Source: CAD feature listing. Evaluate the final solid. Frame: model axes, mm. Face numbers are marked on the shaded views. A direction names the side the tool comes from. Coordinates: 2 decimals unless noted, no trailing zeros. Order: outer loops, then holes, each group sorted by start corner. A loop starts at its lowest first (then second) coordinate and runs counter-clockwise, first axis right, second up.
Item 1: Section A-A on y = 0. Return the cut outline in (x, z).
Item 2: Reachability of the marked faces 1 and 2 from +Z, -Z, +X, -X, +Y, -Y: full face, straight path, thin tool, end or side. Return the list, or none.
Item 3: Mould query, pull axis Y, two halves, no side actions, for the marked faces 3 and 4. Classes: released by +Y, released by -Y, zero draft, split by the parting line, or undercut.
Item 4: Ray query, line 1 (Y direction, x = 2.5, z = 1.25); line 2 (Y direction, x = 0, z = -5.5); line 3 (X direction, y = 6.75, z = 5). Return the intervals inside material, ascending.
Item 5: Contact query for a flat-ended pin moving along its axis: P1, Ø1, axis at y = -1.5, z = -8, coming from the -X side. Output: stop coordinate, or through.
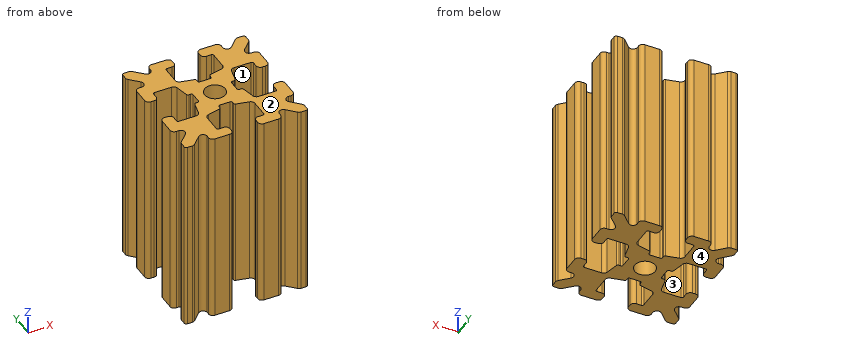
from build123d import *

# Parameters (mm, degrees)
SKETCH1_W           = 15
SKETCH1_H           = 15
SKETCH1_R           = 1.25
BOSS_EXTRUDE1_DEPTH = 12
FILLET1_R           = 0.25
CUT_EXTRUDE1_DEPTH  = 25
CUT_EXTRUDE3_DEPTH  = 25
FILLET3_R           = 0.5
FILLET4_R           = 0.5
FILLET5_R           = 3
FILLET6_R           = 0.2
CUT_EXTRUDE4_DEPTH  = 25
FILLET8_R           = 0.5
SKETCH6_W           = 5.1529354
SKETCH6_H           = 1.651
SKETCH6_W_2         = 1.651
SKETCH6_H_2         = 5.1529354
CUT_EXTRUDE5_DEPTH  = 25
FILLET10_R          = 0.2


with BuildPart() as part:
    # Sketch1 → Boss-Extrude1 (new body, symmetric)
    with BuildSketch(Plane.XY):
        Rectangle(SKETCH1_W, SKETCH1_H)
        Circle(SKETCH1_R, mode=Mode.SUBTRACT)
    extrude(amount=BOSS_EXTRUDE1_DEPTH, both=True)

    # Fillet1
    fillet1_edges = [part.edges().sort_by_distance(p)[0] for p in [
        (7.5, -7.5, 0),
        (-7.5, -7.5, 0),
        (-7.5, 7.5, 0),
        (7.5, 7.5, 0),
    ]]
    fillet(fillet1_edges, radius=FILLET1_R)

    # Sketch2 → Cut-Extrude1 (cut, through all)
    with BuildSketch(Plane.XY.offset(12)):
        Polygon((-7.5, 1.6), (-6.1, 1.6), (-6.1, 2.9), (-3.4, 2.9), (-3.4, -2.9), (-6.1, -2.9), (-6.1, -1.6), (-7.5, -1.6), align=None)
        Polygon((2.9, 6.1), (1.6, 6.1), (1.6, 7.5), (-1.6, 7.5), (-1.6, 6.1), (-2.9, 6.1), (-2.9, 3.4), (2.9, 3.4), align=None)
        Polygon((-1.6, -7.5), (-1.6, -6.1), (-2.9, -6.1), (-2.9, -3.4), (2.9, -3.4), (2.9, -6.1), (1.6, -6.1), (1.6, -7.5), align=None)
        Polygon((6.1, -2.9), (6.1, -1.6), (7.5, -1.6), (7.5, 1.6), (6.1, 1.6), (6.1, 2.9), (3.4, 2.9), (3.4, -2.9), align=None)
    extrude(amount=-CUT_EXTRUDE1_DEPTH, mode=Mode.SUBTRACT)

    # Sketch4 → Cut-Extrude3 (cut, through all)
    with BuildSketch(Plane.XY.offset(12)):
        Polygon((-3.4, 2.9), (-2.75, 0), (-3.4, -2.9), align=None)
        Polygon((-2.9, 3.4), (0, 2.75), (2.9, 3.4), align=None)
        Polygon((3.4, 2.9), (2.75, 0), (3.4, -2.9), align=None)
        Polygon((-2.9, -3.4), (0, -2.75), (2.9, -3.4), align=None)
    extrude(amount=-CUT_EXTRUDE3_DEPTH, mode=Mode.SUBTRACT)

    # Fillet3
    fillet3_edges = [part.edges().sort_by_distance(p)[0] for p in [
        (1.6, -7.5, 0),
        (-1.6, -7.5, 0),
        (-1.6, -6.1, 0),
        (1.6, -6.1, 0),
        (6.1, 1.6, 0),
        (7.5, 1.6, 0),
        (7.5, -1.6, 0),
        (6.1, -1.6, 0),
        (-7.5, -1.6, 0),
        (-7.5, 1.6, 0),
        (-6.1, 1.6, 0),
        (-6.1, -1.6, 0),
        (-1.6, 6.1, 0),
        (-1.6, 7.5, 0),
        (1.6, 7.5, 0),
        (1.6, 6.1, 0),
    ]]
    fillet(fillet3_edges, radius=FILLET3_R)

    # Fillet4
    fillet4_edges = [part.edges().sort_by_distance(p)[0] for p in [
        (-2.9, -3.4, 0),
        (2.9, -3.4, 0),
        (3.4, -2.9, 0),
        (3.4, 2.9, 0),
        (-3.4, 2.9, 0),
        (-3.4, -2.9, 0),
        (2.9, 3.4, 0),
        (-2.9, 3.4, 0),
    ]]
    fillet(fillet4_edges, radius=FILLET4_R)

    # Fillet5
    fillet5_edges = [part.edges().sort_by_distance(p)[0] for p in [
        (-2.75, 0, 0),
        (0, 2.75, 0),
        (2.75, 0, 0),
        (0, -2.75, 0),
    ]]
    fillet(fillet5_edges, radius=FILLET5_R)

    # Fillet6
    fillet6_edges = [part.edges().sort_by_distance(p)[0] for p in [
        (-2.9, -6.1, 0),
        (2.9, -6.1, 0),
        (6.1, -2.9, 0),
        (6.1, 2.9, 0),
        (-6.1, 2.9, 0),
        (-6.1, -2.9, 0),
        (2.9, 6.1, 0),
        (-2.9, 6.1, 0),
    ]]
    fillet(fillet6_edges, radius=FILLET6_R)

    # Sketch5 → Cut-Extrude4 (cut, through all)
    with BuildSketch(Plane.XY.offset(12)):
        Polygon((-7.5, 6.439339828), (-5.460660172, 4.4), (-7.5, 4.4), align=None)
        Polygon((-6.439339828, 7.5), (-4.4, 5.460660172), (-4.4, 7.5), align=None)
        Polygon((4.4, 7.5), (6.439339828, 7.5), (4.4, 5.460660172), align=None)
        Polygon((7.5, 6.439339828), (7.5, 4.4), (5.460660172, 4.4), align=None)
        Polygon((7.5, -6.439339828), (5.460660172, -4.4), (7.5, -4.4), align=None)
        Polygon((6.439339828, -7.5), (4.4, -5.460660172), (4.4, -7.5), align=None)
        Polygon((-4.4, -7.5), (-6.439339828, -7.5), (-4.4, -5.460660172), align=None)
        Polygon((-7.5, -6.439339828), (-7.5, -4.4), (-5.460660172, -4.4), align=None)
    extrude(amount=-CUT_EXTRUDE4_DEPTH, mode=Mode.SUBTRACT)

    # Fillet8
    fillet8_edges = [part.edges().sort_by_distance(p)[0] for p in [
        (-7.5, 4.4, 0),
        (-7.5, 6.439339828, 0),
        (-5.460660172, 4.4, 0),
        (7.5, -4.4, 0),
        (7.5, -6.439339828, 0),
        (5.460660172, -4.4, 0),
        (5.460660172, 4.4, 0),
        (7.5, 6.439339828, 0),
        (7.5, 4.4, 0),
        (-4.4, 7.5, 0),
        (-4.4, 5.460660172, 0),
        (-6.439339828, 7.5, 0),
        (-5.460660172, -4.4, 0),
        (-7.5, -6.439339828, 0),
        (-7.5, -4.4, 0),
        (4.4, 5.460660172, 0),
        (4.4, 7.5, 0),
        (6.439339828, 7.5, 0),
        (6.439339828, -7.5, 0),
        (4.4, -7.5, 0),
        (4.4, -5.460660172, 0),
        (-6.439339828, -7.5, 0),
        (-4.4, -5.460660172, 0),
        (-4.4, -7.5, 0),
    ]]
    fillet(fillet8_edges, radius=FILLET8_R)

    # Sketch6 → Cut-Extrude5 (cut, through all)
    with BuildSketch(Plane.XY.offset(12)):
        with Locations((4.9235323, 0)):
            Rectangle(SKETCH6_W, SKETCH6_H)
        with Locations((0, -4.9235323)):
            Rectangle(SKETCH6_W_2, SKETCH6_H_2)
        with Locations((-4.9235323, 0)):
            Rectangle(SKETCH6_W, SKETCH6_H)
        with Locations((0, 4.9235323)):
            Rectangle(SKETCH6_W_2, SKETCH6_H_2)
    extrude(amount=-CUT_EXTRUDE5_DEPTH, mode=Mode.SUBTRACT)

    # Fillet10
    fillet10_edges = [part.edges().sort_by_distance(p)[0] for p in [
        (0.8255, -2.935025862, 0),
        (-0.8255, -2.935025862, 0),
        (0.8255, -2.3470646, 0),
        (-0.8255, -2.3470646, 0),
        (2.935025862, 0.8255, 0),
        (2.935025862, -0.8255, 0),
        (2.3470646, 0.8255, 0),
        (2.3470646, -0.8255, 0),
        (-2.935025862, -0.8255, 0),
        (-2.935025862, 0.8255, 0),
        (-2.3470646, -0.8255, 0),
        (-2.3470646, 0.8255, 0),
        (-0.8255, 2.935025862, 0),
        (0.8255, 2.935025862, 0),
        (-0.8255, 2.3470646, 0),
        (0.8255, 2.3470646, 0),
    ]]
    fillet(fillet10_edges, radius=FILLET10_R)


solid = part.part
Answer list:
1. outline: (-2.35, -12) - (-1.25, -12) - (-1.25, 12) - (-2.35, 12) - close; (1.25, -12) - (2.35, -12) - (2.35, 12) - (1.25, 12) - close
2. face 1: +Z, -Z
2. face 2: +Z, +X, -X, +Y, -Y
3. face 3: undercut
3. face 4: zero draft
4. line 1: y = -7.5 to -6.1, -3.31 to -0.82, 0.82 to 3.31, 6.1 to 7.5
4. line 2: y = -2.35 to -1.25, 1.25 to 2.35
4. line 3: x = -7.5 to -5.69, -4.4 to -1.6, 1.6 to 4.4, 5.69 to 7.5
5. P1: stops at x = -7.49
